The listing builds one solid part. Answer for the finished solid, in the listing's coordinates (mm). Face numbers are marked on the shaded views. A direction names the side the tool comes from. Coordinates: 2 decimals unless noted, no trailing zeros. Loops run counter-clockwise (first coordinate to the right, second up) from the corner with the lowest first, then second, coordinate; pieces in that order, holes last. Notation, with made-up numbers: M 47,46.5 L 87,46.5 A22 cw 87,79.5 Z; hole C 6,-12 d9. An arc over 180 degrees is marked long. Answer as a JSON object with one key per item and string values. Group by question number.
1. Straight lines are drawn through the part: L1, parallel to Y at x = 8.65, z = 24.05; L2, parallel to X at y = -7, z = 12; L3, parallel to Z at x = 5.5, y = -23.5. For each, find the intervals that lie inside material, in ascending order.
2. A cutting plane is placed at B-B on x = 23.65. Give the vertices of the cut face in (y, z), and give its area (3 significant figures).
3. A cutting plane is placed at C-C on y = -12.1. Give the vertices of the cut face in (x, z).
4. A cutting plane is placed at D-D on z = 2.5. State how many separate pieces and enclosed holes the cut face has, and give its area (3 significant figures).
5. Given pin 1 (1.3 mm diameter, centred on y = -22.72, z = 2, fed in from +X), flat-ended and moving along its own axis, determine where the tip first touches the part or whether it passes through.
6. Determine the mould class of the marked faces 3, 4 and 5 for opening direction X: released by +X, released by -X, zero draft, split by the parting line, or undercut.
7. For the marked faces 1 and 2, determine the directions among +Z, -Z, +X, -X, +Y, -Y from which every point of the face is accessible in a straight line to the end or side of a thin tool.
8. A cutting plane is placed at A-A on z = 11. Give the vertices of the cut face in (x, y).
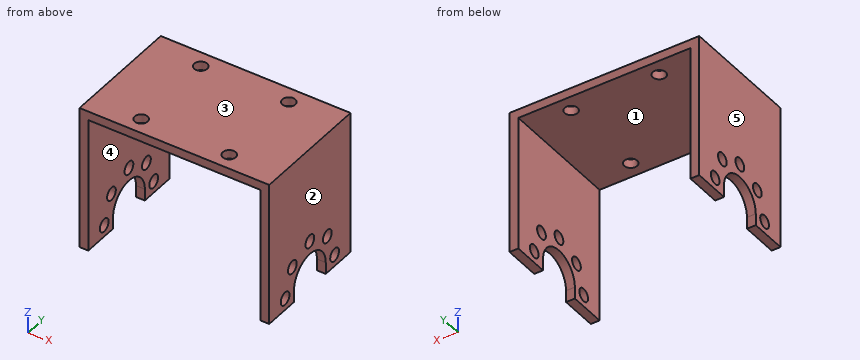
from build123d import *

# Parameters (mm, degrees)
F1_DEPTH = 33
F2_R     = 1.1
F2_W     = 6.27746
F2_H     = 1.5
F3_DEPTH = 32.301
F4_R     = 1.1
F5_DEPTH = 1.5


with BuildPart() as f1:
    # F0 (on Front) → F1 (new body)
    with BuildSketch(Plane.XZ):
        Polygon((0, 24.5), (0, 0), (1.5, 0), (1.5, 23), (30.8, 23), (30.8, 0), (32.3, 0), (32.3, 24.5), align=None)
    extrude(amount=F1_DEPTH)

    # F2 (on face) → F3 (cut, through all)
    with BuildSketch(Plane(origin=(0, 0, 0), x_dir=(0, -1, 0), z_dir=(-1, 0, 0))):
        with BuildLine():
            Line((20.5, 0), (20.5, 2))
            ThreePointArc((20.5, 2), (16.5, 6), (12.5, 2))
            Line((12.5, 2), (12.5, 0))
            Line((12.5, 0), (20.5, 0))
        make_face()
        with Locations((22.72254, 2)):
            Circle(F2_R)
        with Locations((20.9, 6.4)):
            Circle(F2_R)
        with Locations((16.5, 8.22254)):
            Circle(F2_R)
        with Locations((12.1, 6.4)):
            Circle(F2_R)
        with Locations((10.27746, 2)):
            Circle(F2_R)
        Polygon((0, 0), (6.27746, 0), (0, 23), align=None)
        Polygon((0, 23), (6.27746, 0), (6.27746, 23), align=None)
        with Locations((3.13873, 23.75)):
            Rectangle(F2_W, F2_H)
        Polygon((26.72254, 0), (33, 0), (33, 23), align=None)
        Polygon((26.72254, 0), (33, 23), (26.72254, 23), align=None)
        with Locations((29.86127, 23.75)):
            Rectangle(F2_W, F2_H)
    extrude(amount=-F3_DEPTH, mode=Mode.SUBTRACT)

    # F4 (on face) → F5 (cut, through all)
    with BuildSketch(Plane.XY.offset(24.5)):
        with Locations((8.65, -9)):
            Circle(F4_R)
        with Locations((23.65, -9)):
            Circle(F4_R)
        with Locations((8.65, -24)):
            Circle(F4_R)
        with Locations((23.65, -24)):
            Circle(F4_R)
    extrude(amount=-F5_DEPTH, mode=Mode.SUBTRACT)


solid = f1.part
From the geometry:
{
 "1": {"L1": "y = -26.72 to -25.1, -22.9 to -10.1, -7.9 to -6.28", "L2": "x = 0 to 1.5, 30.8 to 32.3", "L3": "z = 23 to 24.5"},
 "2": {"outline": "M -26.72,23 L -25.1,23 L -25.1,24.5 L -26.72,24.5 Z; M -22.9,23 L -10.1,23 L -10.1,24.5 L -22.9,24.5 Z; M -7.9,23 L -6.28,23 L -6.28,24.5 L -7.9,24.5 Z", "area": "24.1 mm²"},
 "3": {"outline": "M 0,0 L 1.5,0 L 1.5,5.3 L 0,5.3 Z; M 0,7.5 L 1.5,7.5 L 1.5,23 L 30.8,23 L 30.8,7.5 L 32.3,7.5 L 32.3,24.5 L 0,24.5 Z; M 30.8,0 L 32.3,0 L 32.3,5.3 L 30.8,5.3 Z"},
 "4": {"separate pieces": "8", "enclosed holes": "0", "area": "25.8 mm²"},
 "5": {"pin 1": "passes through"},
 "6": {"face 3": "zero draft", "face 4": "undercut", "face 5": "released by -X"},
 "7": {"face 1": "-Z, +Y, -Y", "face 2": "+Z, -Z, +X, +Y, -Y"},
 "8": {"outline": "M 0,-26.72 L 1.5,-26.72 L 1.5,-6.28 L 0,-6.28 Z; M 30.8,-26.72 L 32.3,-26.72 L 32.3,-6.28 L 30.8,-6.28 Z"}
}
